For this review, use the dimensioned drawing (mm, ordinates from the lowest corner) and the shaded views. A direction names the side the tool comes from. Give positions to 0.01 mm unless a question says otherwise; leave off trailing zeros. Loops run counter-clockwise (first coordinate to the right, second up) from the corner with the lowest first, then second, coordinate; pieces in that order, holes last. Notation, with made-up numbers: (60.25, -16.5) -> (73.25, -16.5) arc R33 cw to (73.25, 17.5) -> close; hole circle Ø6 at (-22, 25.5). An arc over 180 degrees is marked (long way). Use a Markdown table: item, result. Add a question column.
1. For the marked faces 1 and 2, list the 3-axis set-ups (+Z, -Z, +X, -X, +Y, -Y) from which the entire face can be reached by the end or side of a thin tool; tool diameter is ignored.
2. Add section B-B (y = 39). State the section outline as (x, z) points.
3. Add section A-A (x = 16.25). State the section outline as (y, z) points.
4. Draft analysis for pull direction X (two halves, no side actions). For the marked faces 3, 4 and 5, state which applies: pulls with the +X half, pulls with the -X half, needs draft (parallel to the pull), parting line crosses it, or undercut.
5. Add section D-D (z = 3.45). State the section outline as (x, y) points, and give its area (3 significant figures).
6. Add section C-C (y = 5). State the section outline as (x, z) points, and give its area (3 significant figures).
7. For pin 1 Ø2 at (x, y) = (22.9, 5) entering from +Z, flat-tipped, find the tip position at first contact; note if it passes through.
8. To check wall thickness, follow line 1 (Y direction, x = 8.5, z = 3.5); line 2 (X direction, y = 43, z = 0.7); line 3 (Y direction, x = 7, z = 0.9). State the ranges of each line that lie inside material, in increasing order.
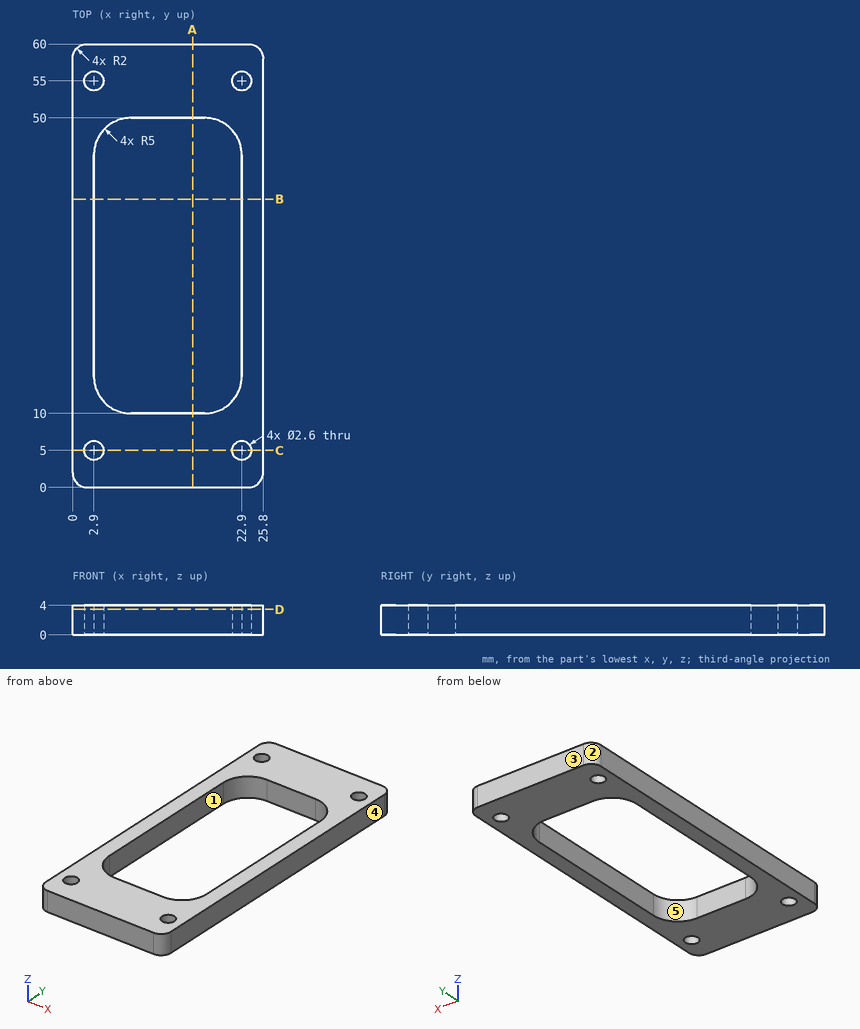
Taken from the geometry:
| question | item | result |
|---|---|---|
| 1 | face 1 | +Z, -Z |
| 1 | face 2 | +Z, -Z, -X, +Y |
| 2 | outline | (0, 0) -> (2.9, 0) -> (2.9, 4) -> (0, 4) -> close; (22.9, 0) -> (25.8, 0) -> (25.8, 4) -> (22.9, 4) -> close |
| 3 | outline | (0, 0) -> (10, 0) -> (10, 4) -> (0, 4) -> close; (50, 0) -> (60, 0) -> (60, 4) -> (50, 4) -> close |
| 4 | face 3 | needs draft |
| 4 | face 4 | pulls with the +X half |
| 4 | face 5 | undercut |
| 5 | outline | (0, 2) arc R2 ccw to (2, 0) -> (23.8, 0) arc R2 ccw to (25.8, 2) -> (25.8, 58) arc R2 ccw to (23.8, 60) -> (2, 60) arc R2 ccw to (0, 58) -> close; hole circle Ø2.6 at (2.9, 5); hole circle Ø2.6 at (2.9, 55); hole (2.9, 15) arc R5 ccw to (7.9, 10) -> (17.9, 10) arc R5 ccw to (22.9, 15) -> (22.9, 45) arc R5 ccw to (17.9, 50) -> (7.9, 50) arc R5 ccw to (2.9, 45) -> close; hole circle Ø2.6 at (22.9, 5); hole circle Ø2.6 at (22.9, 55) |
| 5 | area | 745 mm^2 |
| 6 | outline | (0, 0) -> (1.6, 0) -> (1.6, 4) -> (0, 4) -> close; (4.2, 0) -> (21.6, 0) -> (21.6, 4) -> (4.2, 4) -> close; (24.2, 0) -> (25.8, 0) -> (25.8, 4) -> (24.2, 4) -> close |
| 6 | area | 82.4 mm^2 |
| 7 | pin 1 | passes through |
| 8 | line 1 | y = 0 to 10, 50 to 60 |
| 8 | line 2 | x = 0 to 2.9, 22.9 to 25.8 |
| 8 | line 3 | y = 0 to 10.08, 49.92 to 60 |
